```python
from build123d import *

# Parameters (mm, degrees)
SCHIZZO1_W                   = 6.5
SCHIZZO1_H                   = 40
ESTRUSIONE_ESTRUSIONE1_DEPTH = 2
SCHIZZO2_W                   = 3
SCHIZZO2_H                   = 135
ESTRUSIONE_ESTRUSIONE2_DEPTH = 7
SMUSSO1_SIZE                 = 1
SCHIZZO4_W                   = 3
SCHIZZO4_H                   = 1
TAGLIO_ESTRUSIONE1_DEPTH     = 136.706484738
SMUSSO1_OF_SPECCHIA9_SIZE    = 1


with BuildPart() as part:
    # Schizzo1 → Estrusione-Estrusione1 (new body)
    with BuildSketch(Plane.XY):
        with Locations((3.25, 20)):
            Rectangle(SCHIZZO1_W, SCHIZZO1_H)
    estrusione_estrusione1 = extrude(amount=ESTRUSIONE_ESTRUSIONE1_DEPTH)

    # Schizzo2 → Estrusione-Estrusione2 (add)
    with BuildSketch(Plane(origin=(6.5, 0, 0), x_dir=(0, 0, -1), z_dir=(1, 0, 0))):
        with Locations((-1.5, 20)):
            Rectangle(SCHIZZO2_W, SCHIZZO2_H)
    estrusione_estrusione2 = extrude(amount=ESTRUSIONE_ESTRUSIONE2_DEPTH)

    # Smusso1
    smusso1_edges = [part.edges().sort_by_distance(p)[0] for p in [
        (6.5, 87.5, 1.5),
        (6.5, -47.5, 1.5),
        (13.5, 87.5, 1.5),
        (13.5, -47.5, 1.5),
    ]]
    chamfer(smusso1_edges, length=SMUSSO1_SIZE)

    # Schizzo4 → Taglio-Estrusione1 (cut, through all)
    with BuildSketch(Plane.XZ.offset(47.5)):
        with Locations((10, 2.5)):
            Rectangle(SCHIZZO4_W, SCHIZZO4_H)
    taglio_estrusione1 = extrude(amount=-TAGLIO_ESTRUSIONE1_DEPTH, mode=Mode.SUBTRACT)

    # Specchia9: Estrusione-Estrusione1, Estrusione-Estrusione2, Taglio-Estrusione1 across plane
    add(estrusione_estrusione1.mirror(Plane.ZY))
    add(estrusione_estrusione2.mirror(Plane.ZY))
    add(taglio_estrusione1.mirror(Plane.ZY), mode=Mode.SUBTRACT)

    # Smusso1 of Specchia9
    smusso1_of_specchia9_edges = [part.edges().sort_by_distance(p)[0] for p in [
        (-6.5, 87.5, 1.5),
        (-6.5, -47.5, 1.5),
        (-13.5, 87.5, 1.5),
        (-13.5, -47.5, 1.5),
    ]]
    chamfer(smusso1_of_specchia9_edges, length=SMUSSO1_OF_SPECCHIA9_SIZE)


solid = part.part
```
Geometry: final body of the model. Coordinates: model frame, mm. A direction names the side the tool comes from. Round coordinates to 2 decimals unless told otherwise and drop trailing zeros. Write each loop counter-clockwise with the first axis right and the second up, starting at its lowest first coordinate (ties: lowest second). Pieces come first, ordered by that corner, then holes.
Item 1: Section query A-A (y = -38). Return loops of the section in (x, z), plus the area to 3 significant figures.
Item 2: Section query D-D (x = 9.75). Return loops of the section in (y, z), plus the area to 3 significant figures.
Item 3: Section query C-C (y = 33). Return loops of the section in (x, z).
Item 4: Material intervals for L1, parallel to X at y = -4, z = 2.8; L2, parallel to X at y = 73.5, z = 0.4; L3, parallel to Y at x = 4.5, z = 1.7, sorted ascending.
Item 5: Section query B-B (z = 0.5). Return loops of the section in (x, y).
Item 6: Pin query (flat end, axial travel): P1, Ø12, axis at x = 3, y = -30, coming from the +Z side; P2, Ø6.5, axis at x = -0.5, y = 13, coming from the +Z side; P3, Ø1.6, axis at x = 1.5, z = 0.5, coming from the -Y side. Return the tip coordinate at first contact, or that it passes through.
Item 7: Set-up query: faces 1 (the face through (-10, 19, 2)), 2 (the face through (-6.5, 20.9, 2.2)), 3 (the face through (0, 19, 0)). Return all of +Z, -Z, +X, -X, +Y, -Y with unobstructed straight access to the full face (end or side cutting, diameter ignored); none if empty.
Item 8: Mould query, pull axis X, two halves, no side actions, for faces 4 (the face through (-10, -47.5, 1)), 5 (the face through (-13.5, 21, 2)), 6 (the face through (6.5, 20.9, 2.2)). Classes: +X half, -X half, draft (parallel to the pull), parting line (faces both ways), or undercut.
Completed:
1. outline: (-13.5, 0) - (-6.5, 0) - (-6.5, 3) - (-8.5, 3) - (-8.5, 2) - (-11.5, 2) - (-11.5, 3) - (-13.5, 3) - close; (6.5, 0) - (13.5, 0) - (13.5, 3) - (11.5, 3) - (11.5, 2) - (8.5, 2) - (8.5, 3) - (6.5, 3) - close
1. area: 36.0 mm2
2. outline: (-47.5, 0) - (87.5, 0) - (87.5, 2) - (-47.5, 2) - close
2. area: 270 mm2
3. outline: (-13.5, 0) - (13.5, 0) - (13.5, 3) - (11.5, 3) - (11.5, 2) - (8.5, 2) - (8.5, 3) - (6.5, 3) - (6.5, 2) - (-6.5, 2) - (-6.5, 3) - (-8.5, 3) - (-8.5, 2) - (-11.5, 2) - (-11.5, 3) - (-13.5, 3) - close
4. L1: x = -13.5 to -11.5, -8.5 to -6.5, 6.5 to 8.5, 11.5 to 13.5
4. L2: x = -13.5 to -6.5, 6.5 to 13.5
4. L3: y = 0 to 40
5. outline: (-13.5, -46.5) - (-12.5, -47.5) - (-7.5, -47.5) - (-6.5, -46.5) - (-6.5, 0) - (6.5, 0) - (6.5, -46.5) - (7.5, -47.5) - (12.5, -47.5) - (13.5, -46.5) - (13.5, 86.5) - (12.5, 87.5) - (7.5, 87.5) - (6.5, 86.5) - (6.5, 40) - (-6.5, 40) - (-6.5, 86.5) - (-7.5, 87.5) - (-12.5, 87.5) - (-13.5, 86.5) - close
6. P1: stops at z = 3
6. P2: stops at z = 2
6. P3: stops at y = 0
7. face 1: +Z, +Y, -Y
7. face 2: +Z
7. face 3: -Z, +X, -X, +Y, -Y
8. face 4: draft
8. face 5: -X half
8. face 6: undercut
